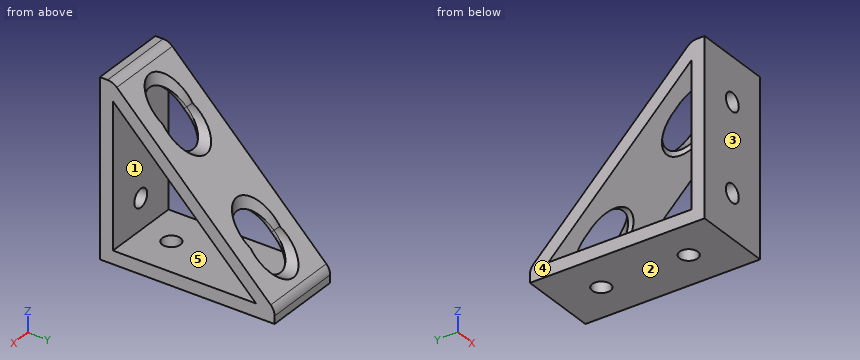
Autodesk Inventor part; units mm, degrees
ref_plane "YZ Plane" through (0, 0, 0) normal (1, 0, 0) x (0, 1, 0)
ref_plane "XZ Plane" through (0, 0, 0) normal (0, 1, 0) x (-1, 0, 0)
ref_plane "XY Plane" through (0, 0, 0) normal (0, 0, 1) x (1, 0, 0)
sketch "Sketch_1" plane through (0, 0, 0) normal (1, 0, 0) x (0, 1, 0)
  line L0 (3.5147, 80) -> (0, 80)
  line L1 (0, 80) -> (0, 0)
  line L2 (0, 0) -> (80, 0)
  line L3 (80, 0) -> (80, 3.5147)
  arc A0 (80, 3.5147) -> (78.2426, 7.7574) centre (74, 3.5147) ccw
  line L4 (78.2426, 7.7574) -> (7.7574, 78.2426)
  arc A1 (7.7574, 78.2426) -> (3.5147, 80) centre (3.5147, 74) ccw
  line L5 (6, 71.5147) -> (6, 6)
  line L6 (6, 6) -> (71.5147, 6)
  line L7 (71.5147, 6) -> (6, 71.5147)
extrude "Extrusion1" add sketch "Sketch_1" along normal mid plane 36
sketch "Sketch2" plane through (-18, 0, 0) normal (0, -1, 0) x (1, 0, 0)
  point P0 (18, 20)
hole "Hole1" at (0, 0, 20) direction (0, 1, 0) diameter 8.33 depth 6
sketch "Sketch3" plane through (18, 80, 0) normal (0, 0, -1) x (-1, 0, 0)
  point P0 (18, -60)
hole "Hole2" at (0, 20, 0) direction (0, 0, 1) diameter 8.33 depth 6
sketch "Sketch_4" plane through (0, 0, 80) normal (0, 0, 1) x (1, 0, 0)
  circle A0 centre (0, 20) radius 10
extrude "Extrusion2" cut sketch "Sketch_4" against normal blind 74
sketch "Sketch_5" plane through (0, 80, 0) normal (0, 1, 0) x (1, 0, 0)
  circle A0 centre (0, -20) radius 10
extrude "Extrusion3" cut sketch "Sketch_5" against normal blind 74
sketch "Sketch6" plane through (18, 80, 0) normal (0, 0, -1) x (-1, 0, 0)
  point P0 (18, -20)
hole "Hole3" at (0, 60, 0) direction (0, 0, 1) diameter 8.33 depth 6
sketch "Sketch7" plane through (-18, 0, 0) normal (0, -1, 0) x (1, 0, 0)
  point P0 (18, 60)
hole "Hole4" at (0, 0, 60) direction (0, 1, 0) diameter 8.33 depth 6
sketch "Sketch_8" plane through (0, 0, 80) normal (0, 0, 1) x (1, 0, 0)
  circle A0 centre (0, 60) radius 10
extrude "Extrusion4" cut sketch "Sketch_8" against normal blind 74
sketch "Sketch_9" plane through (0, 80, 0) normal (0, 1, 0) x (1, 0, 0)
  circle A0 centre (0, -60) radius 10
extrude "Extrusion5" cut sketch "Sketch_9" against normal blind 74
properties part number "40-4336 Aluminum"
The listing builds one solid part. Answer for the finished solid, in the listing's coordinates (mm). Face numbers are marked on the shaded views. A direction names the side the tool comes from. Give positions to 0.01 mm unless a question says otherwise; leave off trailing zeros. Loops run counter-clockwise (first coordinate to the right, second up) from the corner with the lowest first, then second, coordinate; pieces in that order, holes last. Notation, with made-up numbers: (14.5, 58.25) - (37.5, 58.25) arc R31 ccw to (37.5, 90.25) - close; hole circle Ø9 at (32, -0.5). An arc over 180 degrees is marked (long way). Return JSON: item names as keys, results as strings. Group by question number.
1. Straight lines are drawn through the part: line 1 (Z direction, x = 0, y = 3.2) (3 decimals); line 2 (Y direction, x = 0, z = 3.9) (3 decimals); line 3 (X direction, y = 60, z = 4.65) (3 decimals). For each, find the intervals that lie inside material, in ascending order. Write a range as [from, to].
2. Determine the mould class of the marked faces 3, 4 and 5 for opening direction Y: pulls with the +Y half, pulls with the -Y half, needs draft (parallel to the pull), parting line crosses it, or undercut.
3. Find section C-C (x = 0). State how many separate pieces and enclosed holes the cut face has, then the cut area to 3 significant figures.
4. Given pin 1 Ø11 at (x, z) = (0, 20) entering from +Y; pin 2 Ø6 at (x, z) = (-11, 31) entering from +Y; pin 3 Ø11 at (x, y) = (-1.5, 22.5) entering from +Z, each flat-ended and moving along its own axis, determine where each tip first touches the part or whether it passes through.
5. Which of the six approach directions +Z, -Z, +X, -X, +Y, -Y give full straight-line access (tool end or side, diameter ignored) to the marked faces 1 and 2?
6. Find section A-A (x = 13). Write down the section's boundary in (y, z), then the cut area to 3 significant figures.
7. Find section B-B (z = 44). Write down the section's boundary in (x, y).
8. Find section D-D (y = 37). Write down the section's boundary in (x, z), then the cut area to 3 significant figures.
Verdict:
{
 "1": {"line 1": "z = [0, 15.835], [24.165, 55.835], [64.165, 80]", "line 2": "y = [0, 15.835], [24.165, 55.835], [64.165, 79.988]", "line 3": "x = [-18, -4.165], [4.165, 18]"},
 "2": {"face 3": "pulls with the -Y half", "face 4": "needs draft", "face 5": "undercut"},
 "3": {"separate pieces": "6", "enclosed holes": "0", "area": "933 mm^2"},
 "4": {"pin 1": "stops at y = 6", "pin 2": "stops at y = 58", "pin 3": "stops at z = 6"},
 "5": {"face 1": "+X, -X", "face 2": "-Z, +X, -X, +Y, -Y"},
 "6": {"outline": "(0, 0) - (80, 0) - (80, 3.51) arc R6 ccw to (78.24, 7.76) - (7.76, 78.24) arc R6 ccw to (3.51, 80) - (0, 80) - close; hole (6, 6) - (71.51, 6) - (6, 71.51) - close", "area": "1,510 mm^2"},
 "7": {"outline": "(-18, 0) - (18, 0) - (18, 6) - (-18, 6) - close; (-18, 33.51) - (18, 33.51) - (18, 42) - (-18, 42) - close"},
 "8": {"outline": "(-18, 0) - (18, 0) - (18, 6) - (-18, 6) - close; (-18, 40.51) - (18, 40.51) - (18, 49) - (-18, 49) - close", "area": "521 mm^2"}
}
